Verification items for this drawing (mm, ordinates from the low corner). A direction names the side the tool comes from. Coordinates: 2 decimals unless noted, no trailing zeros. Order: outer loops, then holes, each group sorted by start corner. A loop starts at its lowest first (then second) coordinate and runs counter-clockwise, first axis right, second up. Notation, with made-up numbers: (23.5, 47) -> (60.5, 47) arc R30 cw to (60.5, 84) -> close; hole circle Ø3 at (42.5, 11.5). An arc over 180 degrees is marked (long way). Write item = value, one per line. Start each with the question number.
1. Set-up check for the marked faces 1 and 2: record each of +Z, -Z, +X, -X, +Y, -Y from which the full face is reachable in a straight line by a thin tool's end or side.
2. Cross-section at A-A on z = 3.5. Record the cut outline in (x, y), plus the area to 3 significant figures.
3. Go/stop test with a flat-tipped pin: P1, Ø1.8, axis at x = 27, y = 27, coming from the -Z side. Record where the tip stops, or that it passes through.
4. Cross-section at B-B on y = 16.5. Record the cut outline in (x, z).
5. Thickness scan on line 1 along Y through (x, z) = (3, 5.25); line 2 along Y through (x, z) = (3.5, 10.25); line 3 along X through (y, z) = (15, 8). Record the ranges inside material, lowest first. Write a range as from..to.
6. Cross-section at D-D on x = 12.25. Record the cut outline in (y, z).
7. Cross-section at C-C on x = 16.5. Record the cut outline in (y, z).
8. Release check for a two-part mould opening along X. For the marked faces 3, 4 and 5 record: +X half, -X half, draft (parallel to the pull), parting line (faces both ways), or undercut.
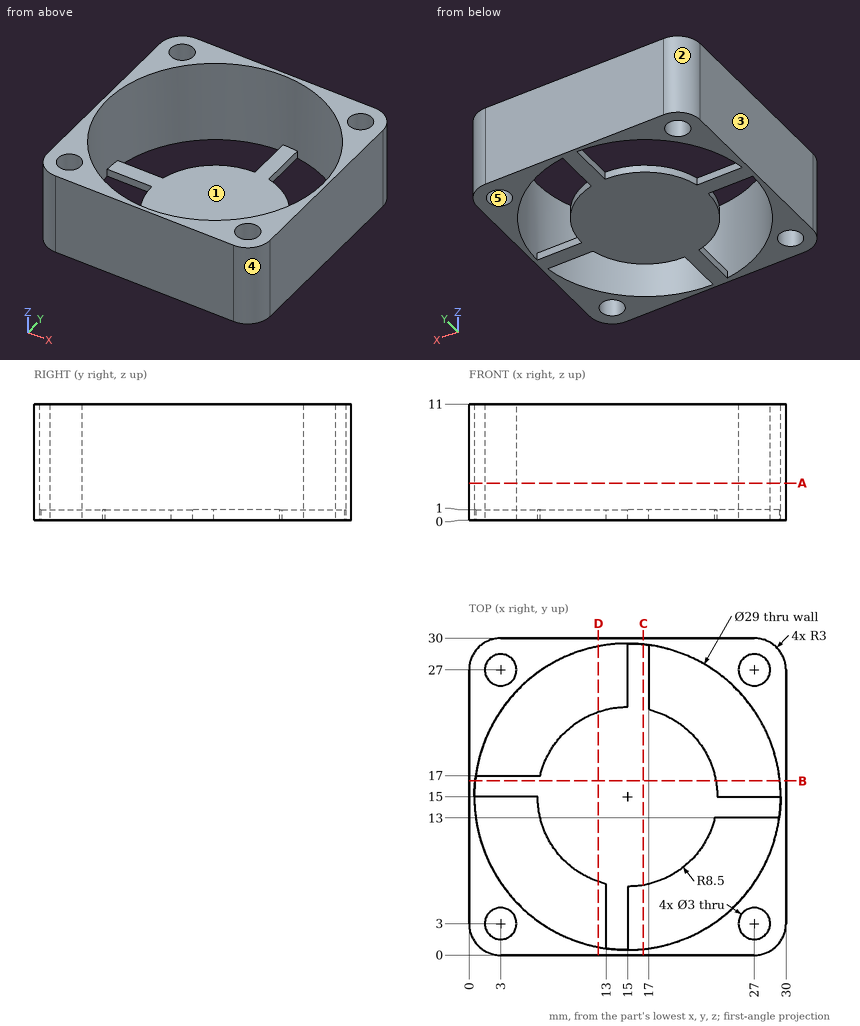
Worked out:
q1.face_1 = +Z
q1.face_2 = +Z, -Z, -X, +Y
q2.outline = (0, 3) arc R3 ccw to (3, 0) -> (27, 0) arc R3 ccw to (30, 3) -> (30, 27) arc R3 ccw to (27, 30) -> (3, 30) arc R3 ccw to (0, 27) -> close; hole circle Ø29 at (15, 15); hole circle Ø3 at (3, 3); hole circle Ø3 at (3, 27); hole circle Ø3 at (27, 3); hole circle Ø3 at (27, 27)
q2.area = 203 mm²
q3.P1 = through
q4.outline = (0, 0) -> (23.37, 0) -> (23.37, 1) -> (0.58, 1) -> (0.58, 11) -> (0, 11) -> close; (29.42, 0) -> (30, 0) -> (30, 11) -> (29.42, 11) -> close
q5.line_1 = 0..1.5, 4.5..6.86, 23.14..25.5, 28.5..30
q5.line_2 = 0..1.59, 4.41..6.17, 23.83..25.59, 28.41..30
q5.line_3 = 0..0.5, 29.5..30
q6.outline = (0, 0) -> (0.76, 0) -> (0.76, 11) -> (0, 11) -> close; (6.96, 0) -> (23.04, 0) -> (23.04, 1) -> (6.96, 1) -> close; (29.24, 0) -> (30, 0) -> (30, 11) -> (29.24, 11) -> close
q7.outline = (0, 0) -> (0.58, 0) -> (0.58, 11) -> (0, 11) -> close; (6.63, 0) -> (30, 0) -> (30, 11) -> (29.42, 11) -> (29.42, 1) -> (6.63, 1) -> close
q8.face_3 = -X half
q8.face_4 = +X half
q8.face_5 = undercut
